For this review, take the finished solid that the model builds, in its own axes (mm). Face numbers are marked on the shaded views. Round coordinates to 2 decimals unless told otherwise and drop trailing zeros. Order: outer loops, then holes, each group sorted by start corner. A loop starts at its lowest first (then second) coordinate and runs counter-clockwise, first axis right, second up. Notation, with made-up numbers: M 53,53 L 60,53 A29 cw 60,86 Z; hole C 81.5,48.25 d8. An arc over 180 degrees is marked long. Answer as a JSON object with one key per item and string values.
from build123d import *

# Parameters (mm, degrees)
BOSS_EXTRUDE1_DEPTH      = 5
BOSS_EXTRUDE1_DEPTH_BACK = 5
SKETCH2_R                = 1.55


with BuildPart() as part:
    # Sketch2 → Boss-Extrude1 (new, two sides: drawn at the far end of the back side and taken through both)
    with BuildSketch(Plane.XY.offset(-BOSS_EXTRUDE1_DEPTH_BACK)):
        with BuildLine():
            Line((2.905523423, 2.749169627), (-11.641714865, 18.12375444))
            ThreePointArc((-11.641714865, 18.12375444), (-18.21926668, 19.574482524), (-22, 14))
            ThreePointArc((-22, 14), (-42.474078457, 23.622085), (-60.163399658, 37.723869421))
            ThreePointArc((-60.163399658, 37.723869421), (-76.495910352, 60.486816081), (-80.043672644, 88.277390543))
            ThreePointArc((-80.043672644, 88.277390543), (-85.99568578, 94.999998449), (-91.957360362, 88.285956923))
            ThreePointArc((-91.957360362, 88.285956923), (-84.145355247, 58.049091263), (-68.630234445, 30.946019566))
            ThreePointArc((-68.630234445, 30.946019566), (-38.101001964, 6.292742427), (-0.232587209, -3.993232173))
            ThreePointArc((-0.232587209, -3.993232173), (3.626450401, -1.687855885), (2.905523423, 2.749169627))
        make_face()
        with Locations((-86, 89)):
            Circle(SKETCH2_R, mode=Mode.SUBTRACT)
        with Locations((-16, 14)):
            Circle(SKETCH2_R, mode=Mode.SUBTRACT)
        with Locations((-3.6022, 2.7054)):
            Circle(SKETCH2_R, mode=Mode.SUBTRACT)
    extrude(amount=BOSS_EXTRUDE1_DEPTH + BOSS_EXTRUDE1_DEPTH_BACK)


solid = part.part
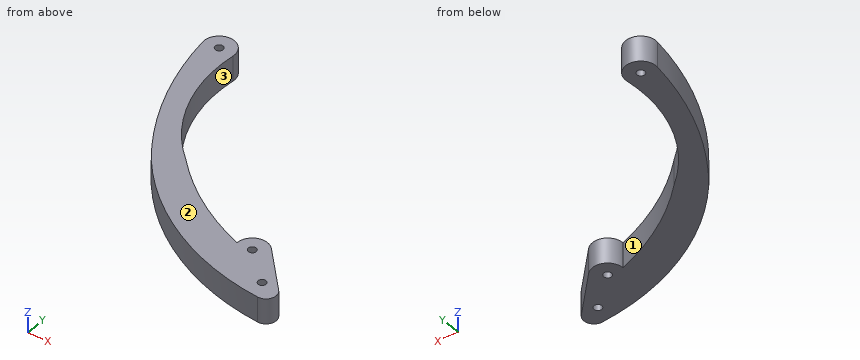
1) Insertion check: P1, Ø4, axis at x = -39.5, z = 1, coming from the +Y side; P2, Ø5, axis at y = 42.5, z = 0.5, coming from the -X side; P3, Ø2, axis at y = 6.5, z = 2.5, coming from the +X side. Each pin has a flat end and moves straight along its axis. Give the tip position at first contact, or say it passes through.
Geometry check:
{"P1": "stops at y = 23.02", "P2": "stops at x = -77.87", "P3": "stops at x = 0.3"}
2) Mouldability with a two-part tool opening along X and no side actions: class the marked faces 1, 2 and 3 as +X half, -X half, draft (parallel to the pull), parting line (faces both ways), or undercut.
Geometry check:
{"face 1": "undercut", "face 2": "draft", "face 3": "+X half"}
3) Add section B-B on z = -2.25. State the section outline as (x, y) points.
Geometry check:
{"outline": "M -91.96,88.29 A117.28 ccw -68.63,30.95 A95.44 ccw -0.23,-3.99 A4 ccw 2.91,2.75 L -11.64,18.12 A6 ccw -22,14 A97.02 cw -60.16,37.72 A57.13 cw -80.04,88.28 A6 ccw long Z; hole C -86,89 d3.1; hole C -16,14 d3.1; hole C -3.6,2.71 d3.1"}
4) Add section C-C on x = -16. State the section outline as (y, z) points, and give its area (3 significant figures).
Geometry check:
{"outline": "M -1.74,-5 L 12.45,-5 L 12.45,5 L -1.74,5 Z; M 15.55,-5 L 20,-5 L 20,5 L 15.55,5 Z", "area": "186 mm²"}
5) For L1, parallel to X at y = 89, z = 0.5; L2, parallel to Y at x = -15, z = -3.75; L3, parallel to Y at x = -16, z = -0.75, list the stretches that pass through material, from the lowest coordinate up.
Geometry check:
{"L1": "x = -92 to -87.55, -84.45 to -80", "L2": "y = -1.97 to 12.82, 15.18 to 19.92", "L3": "y = -1.74 to 12.45, 15.55 to 20"}
6) Add section A-A on x = -86. State the section outline as (y, z) points.
Geometry check:
{"outline": "M 62.91,-5 L 87.45,-5 L 87.45,5 L 62.91,5 Z; M 90.55,-5 L 95,-5 L 95,5 L 90.55,5 Z"}
7) Add section D-D on x = -66.5. State the section outline as (y, z) points.
Geometry check:
{"outline": "M 28.43,-5 L 43.98,-5 L 43.98,5 L 28.43,5 Z"}
